from build123d import *

# Parameters (mm, degrees)
SKETCH1_W            = 42
SKETCH1_H            = 20.5
BOSS_EXTRUDE1_DEPTH  = 39.5
BOSS_EXTRUDE2_START  = -0.5
SKETCH2_W            = 56
SKETCH2_H            = 2.5
BOSS_EXTRUDE2_DEPTH  = 19.5
CUT_EXTRUDE1_DEPTH   = 40
MIRROR2_COPY_1_DEPTH = 40
CUT_EXTRUDE2_DEPTH   = 40
SKETCH5_R            = 3
BOSS_EXTRUDE3_DEPTH  = 6
SKETCH6_R            = 6.75
BOSS_EXTRUDE4_DEPTH  = 2
SKETCH7_R            = 1.15
CUT_EXTRUDE3_DEPTH   = 5
FILLET1_R            = 0.5
SKETCH8_W            = 6.2
SKETCH8_H            = 4
BOSS_EXTRUDE5_DEPTH  = 5.5
BOSS_EXTRUDE5_TAPER  = 5
CHAMFER1_SIZE        = 1


with BuildPart() as part:
    # Sketch1 → Boss-Extrude1 (new body)
    with BuildSketch(Plane(origin=(0, 0, 0), x_dir=(1, 0, 0), z_dir=(0, 1, 0))):
        Rectangle(SKETCH1_W, SKETCH1_H)
    extrude(amount=BOSS_EXTRUDE1_DEPTH)

    # Sketch2 → Boss-Extrude2 (add)
    with BuildSketch(Plane.XY.offset(10.25).offset(BOSS_EXTRUDE2_START)):
        with Locations((0, 29.75)):
            Rectangle(SKETCH2_W, SKETCH2_H)
    extrude(amount=-BOSS_EXTRUDE2_DEPTH)

    # Sketch3 → Cut-Extrude1 (cut)
    with BuildSketch(Plane(origin=(0, 31, 0), x_dir=(1, 0, 0), z_dir=(0, 1, 0))):
        with BuildLine():
            Line((26.370828693, 3.75), (28, 3.75))
            Line((28, 3.75), (28, 6.25))
            Line((28, 6.25), (26.370828693, 6.25))
            ThreePointArc((26.370828693, 6.25), (22.25, 5), (26.370828693, 3.75))
        make_face()
    cut_extrude1 = extrude(amount=-CUT_EXTRUDE1_DEPTH, mode=Mode.SUBTRACT)

    # Mirror1: Cut-Extrude1 across plane
    add(cut_extrude1.mirror(Plane.XY), mode=Mode.SUBTRACT)

    # Mirror2: Cut-Extrude1 across plane
    add(cut_extrude1.mirror(Plane(origin=(0, 0, 0), x_dir=(0, 0, 1), z_dir=(1, 0, 0))), mode=Mode.SUBTRACT)

    # Mirror2 copy 1 sketch → Mirror2 copy 1 (cut)
    with BuildSketch(Plane(origin=(0, 31, 0), x_dir=(-1, 0, 0), z_dir=(0, 1, 0))):
        with BuildLine():
            Line((26.370828693, 3.75), (28, 3.75))
            Line((28, 3.75), (28, 6.25))
            Line((28, 6.25), (26.370828693, 6.25))
            ThreePointArc((26.370828693, 6.25), (22.25, 5), (26.370828693, 3.75))
        make_face()
    extrude(amount=-MIRROR2_COPY_1_DEPTH, mode=Mode.SUBTRACT)

    # Sketch4 → Cut-Extrude2 (cut)
    with BuildSketch(Plane.XY.offset(10.25)):
        Polygon((-21, 34.5), (-12.5, 39.5), (-12.5, 42.326326537), (-24.476884638, 42.326326537), (-24.476884638, 34.5), align=None)
    extrude(amount=-CUT_EXTRUDE2_DEPTH, mode=Mode.SUBTRACT)

    # Sketch5 → Boss-Extrude3 (add)
    with BuildSketch(Plane(origin=(0, 39.5, 0), x_dir=(1, 0, 0), z_dir=(0, 1, 0))):
        with Locations(Location((10.5, 0, 0), (0, 0, 90))):
            Circle(SKETCH5_R)
    extrude(amount=BOSS_EXTRUDE3_DEPTH)

    # Sketch6 → Boss-Extrude4 (add)
    with BuildSketch(Plane(origin=(0, 39.5, 0), x_dir=(1, 0, 0), z_dir=(0, 1, 0))):
        with Locations(Location((10.5, 0, 0), (0, 0, 90))):
            Circle(SKETCH6_R)
    extrude(amount=BOSS_EXTRUDE4_DEPTH)

    # Sketch7 → Cut-Extrude3 (cut)
    with BuildSketch(Plane(origin=(0, 45.5, 0), x_dir=(1, 0, 0), z_dir=(0, 1, 0))):
        with Locations(Location((10.5, 0, 0), (0, 0, 270))):
            Circle(SKETCH7_R)
    extrude(amount=-CUT_EXTRUDE3_DEPTH, mode=Mode.SUBTRACT)

    # Fillet1
    fillet1_edges = [part.edges().sort_by_distance(p)[0] for p in [
        (-21, 17.25, -10.25),
        (-21, 17.25, 10.25),
        (21, 19.75, -10.25),
        (21, 19.75, 10.25),
    ]]
    fillet(fillet1_edges, radius=FILLET1_R - 0.0001)  # a hair under: the kernel refuses the full size

    # Sketch8 → Boss-Extrude5 (add)
    with BuildSketch(Plane(origin=(21, 0, 0), x_dir=(0, 0, -1), z_dir=(1, 0, 0))):
        with Locations((0, 6.6)):
            Rectangle(SKETCH8_W, SKETCH8_H)
    extrude(amount=BOSS_EXTRUDE5_DEPTH, taper=BOSS_EXTRUDE5_TAPER)

    # Chamfer1
    chamfer1_edges = [part.edges().sort_by_distance(p)[0] for p in [
        (10.5, 41.5, 6.75),
    ]]
    chamfer(chamfer1_edges, length=CHAMFER1_SIZE)


solid = part.part
CAD build for the part. Positions are in the model's coordinates, mm. A direction names the side the tool comes from. Round coordinates to 2 decimals unless told otherwise and drop trailing zeros. Write each loop counter-clockwise with the first axis right and the second up, starting at its lowest first coordinate (ties: lowest second). Pieces come first, ordered by that corner, then holes.
(1) 3-axis set-ups, long thin cutter, end or side, ignore diameter. For faces 1 (the face through (27, 30, 6.25)), 2 (the face through (-25, 31, 0)), 3 (the face through (-21, 17, 0)), 4 (the face through (24, 28.5, 0)), 5 (the face through (16.49, 39.99, -3.11)): which of +Z, -Z, +X, -X, +Y, -Y reach the whole face in a straight line?
(2) Slice it at C-C, the plane z = -8.5. Write the cut outline in (x, y), and give its area (3 significant figures).
(3) Slice it at D-D, the plane x = 10.5. Write the cut outline in (y, z).
(4) Probe line 1 along Z through (x, y) = (-24.5, 30.55); line 2 along X through (y, z) = (18.5, 4.25); line 3 along X through (y, z) = (43.85, 0). List the from-to ranges inside material, lowest first.
(5) Slice it at B-B, the plane y = 15. Write the cut outline in (x, z), and give its area (3 significant figures).
(6) Mould opens along Y. For faces 6 (the face through (21, 19, 0)), 7 (the face through (12, 45.5, 0)), 8 (the face through (27, 30, -6.25)) say: pulls with the +Y half, pulls with the -Y half, needs draft (parallel to the pull), parting line crosses it, or undercut.
(7) Drop flat-ended pins along their axis: P1, Ø3, axis at x = -26, y = 30, coming from the +Z side; P2, Ø0.8, axis at x = 26, y = 29.5, coming from the -Z side; P3, Ø7.5, axis at x = -24, z = 3, coming from the -Y side; P4, Ø0.7, axis at x = 11, z = -0.5, coming from the +Y side. Give the stop position or say it passes through.
(8) Slice it at A-A, the plane x = -24.5. Write the cut outline in (y, z), and give its area (4 significant figures).
From the geometry:
1. face 1: +X, +Y, -Y
1. face 2: +Z, -Z, -X, +Y
1. face 3: +Z, -Z, -X
1. face 4: +Z, -Z, +X
1. face 5: +Y
2. outline: (-28, 28.5) - (-21, 28.5) - (-21, 0) - (21, 0) - (21, 28.5) - (28, 28.5) - (28, 31) - (21, 31) - (21, 39.5) - (-12.5, 39.5) - (-21, 34.5) - (-21, 31) - (-28, 31) - close
2. area: 1,670 mm2
3. outline: (0, -10.25) - (39.5, -10.25) - (39.5, -6.75) - (40.5, -6.75) - (41.5, -5.75) - (41.5, -3) - (45.5, -3) - (45.5, -1.15) - (40.5, -1.15) - (40.5, 1.15) - (45.5, 1.15) - (45.5, 3) - (41.5, 3) - (41.5, 5.75) - (40.5, 6.75) - (39.5, 6.75) - (39.5, 10.25) - (0, 10.25) - close
4. line 1: z = -9.75 to -7.25, -2.75 to 2.75, 7.25 to 9.75
4. line 2: x = -21 to 21
4. line 3: x = 7.5 to 9.35, 11.65 to 13.5
5. outline: (-21, -9.75) arc R0.5 ccw to (-20.5, -10.25) - (20.5, -10.25) arc R0.5 ccw to (21, -9.75) - (21, 9.75) arc R0.5 ccw to (20.5, 10.25) - (-20.5, 10.25) arc R0.5 ccw to (-21, 9.75) - close
5. area: 861 mm2
6. face 6: undercut
6. face 7: pulls with the +Y half
6. face 8: needs draft
7. P1: stops at z = 9.75
7. P2: stops at z = -9.75
7. P3: stops at y = 0
7. P4: stops at y = 40.5
8. outline: (28.5, -9.75) - (31, -9.75) - (31, -7.25) - (28.5, -7.25) - close; (28.5, -2.75) - (31, -2.75) - (31, 2.75) - (28.5, 2.75) - close; (28.5, 7.25) - (31, 7.25) - (31, 9.75) - (28.5, 9.75) - close
8. area: 26.25 mm2
